Here's how the part is built. I have some questions about the finished solid (model axes, mm). A direction names the side the tool comes from. Coordinates: 2 decimals unless noted, no trailing zeros. Write each loop counter-clockwise with the first axis right and the second up, starting at its lowest first coordinate (ties: lowest second). Pieces come first, ordered by that corner, then holes.
```python
from build123d import *

# Parameters (mm, degrees)
CONG_1_R                     = 1
CHANFREIN1_SIZE              = 0.5
R_P_TITION_CIRCULAIRE1_COUNT = 4


with BuildPart() as part:
    # Esquisse1 → Révolution1 (revolve)
    with BuildSketch(Plane.XY, mode=Mode.PRIVATE) as r_volution1_sk:
        Polygon((81.575845111, 40), (95.575845111, 40), (95.575845111, 60), (109.575845111, 60), (109.575845111, 34), (81.575845111, 34), align=None)
    revolve(r_volution1_sk.sketch.rotate(Axis((0, 0, 0), (1, 0, 0)), 90), axis=Axis((0, 0, 0), (1, 0, 0)))

    # Congé1
    cong_1_edges = [part.edges().sort_by_distance(p)[0] for p in [
        (109.575845111, 0, -60),
    ]]
    fillet(cong_1_edges, radius=CONG_1_R)

    # Chanfrein1
    chanfrein1_edges = [part.edges().sort_by_distance(p)[0] for p in [
        (81.575845111, 0, -40),
    ]]
    chamfer(chanfrein1_edges, length=CHANFREIN1_SIZE)

    # Esquisse6 → Chambrage pour vis à six pans creux M81 (revolve, cut)
    with BuildSketch(Plane(origin=(109.575845111, 50, 0), x_dir=(0, 0, -1), z_dir=(0, 1, 0))):
        Polygon((0, 0), (0, 28), (4.5, 28), (4.5, 8.6), (7.5, 8.6), (7.5, 0.025), (7.525, 0), align=None)
    chambrage_pour_vis_six_pans_creux_m81 = revolve(axis=Axis((115.925845111, 50, 0), (-1, 0, 0)), mode=Mode.SUBTRACT)

    # Répétition circulaire1: Chambrage pour vis à six pans creux M81 ×4 about axis
    r_p_tition_circulaire1_axis = Axis((0, 0, 0), (1, 0, 0))
    for i in range(1, R_P_TITION_CIRCULAIRE1_COUNT):
        add(chambrage_pour_vis_six_pans_creux_m81.rotate(r_p_tition_circulaire1_axis, i * 360 / R_P_TITION_CIRCULAIRE1_COUNT), mode=Mode.SUBTRACT)


solid = part.part
```
1) On a 3-axis mill with a long thin cutter (end or side, diameter ignored), from which of +Z, -Z, +X, -X, +Y, -Y can I reach the whole of each face in a straight line? I mean faces 4 (the face through (109.576, 25, 25)), 5 (the face through (100.976, 5, -50)). Say none if no direction works.
Values follow:
face 4: +Z, -Z, +X, +Y, -Y
face 5: +X
2) Will these pins go through, and if not, where does the flat tip stop? pin 1 (7.5 mm diameter, centred on y = -52.5, z = -3.5, fed in from +X); pin 2 (10 mm diameter, centred on x = 103, y = 17.5, fed in from -Z); pin 3 (13.5 mm diameter, centred on y = -50, z = 0, fed in from -X); pin 4 (2 mm diameter, centred on x = 101.5, y = 8, fed in from +Z).
Values follow:
pin 1: stops at x = 109.58
pin 2: stops at z = -58.68
pin 3: stops at x = 95.58
pin 4: stops at z = 59.59
3) Imagine slicing it at C-C on x = 93. Please give me the cut outline in (y, z), then the cut area to 3 significant figures.
Values follow:
outline: circle Ø80 at (0, 0); hole circle Ø68 at (0, 0)
area: 1,390 mm2
4) Imagine slicing it at B-B on y = 0. Count the separate pieces of the cut face and the enclosed holes in it, then the cut area to 3 significant figures.
Values follow:
separate pieces: 4
enclosed holes: 0
area: 540 mm2
5) I need wall thicknesses on probe 1 along Y at (x, z) = (99.5, 0); probe 2 along Y at (x, z) = (103.5, 0); probe 3 along X at (y, z) = (-28.5, 31). Which ranges of each line are inside material? Lowest first, please.
Values follow:
probe 1: y = -60 to -54.5, -45.5 to -34, 34 to 45.5, 54.5 to 60
probe 2: y = -60 to -57.5, -42.5 to -34, 34 to 42.5, 57.5 to 60
probe 3: x = 95.58 to 109.58
6) We'd pull the mould along Z, two halves only. Please class faces 1 (the face through (88.92, -1.76, -39.96)), 2 (the face through (81.576, -29.4, -17.4)), 3 (the face through (105.32, 1.63, -57.32)): pulls with the +Z half, pulls with the -Z half, needs draft (parallel to the pull), parting line crosses it, or undercut.
Values follow:
face 1: parting line crosses it
face 2: needs draft
face 3: undercut
7) Imagine slicing it at A-A on x = 102.5. Please give me the cut outline in (y, z), then the cut area to 3 significant figures.
Values follow:
outline: circle Ø120 at (0, 0); hole circle Ø15 at (-50, 0); hole circle Ø68 at (0, 0); hole circle Ø15 at (0, -50); hole circle Ø15 at (0, 50); hole circle Ø15 at (50, 0)
area: 6,970 mm2
